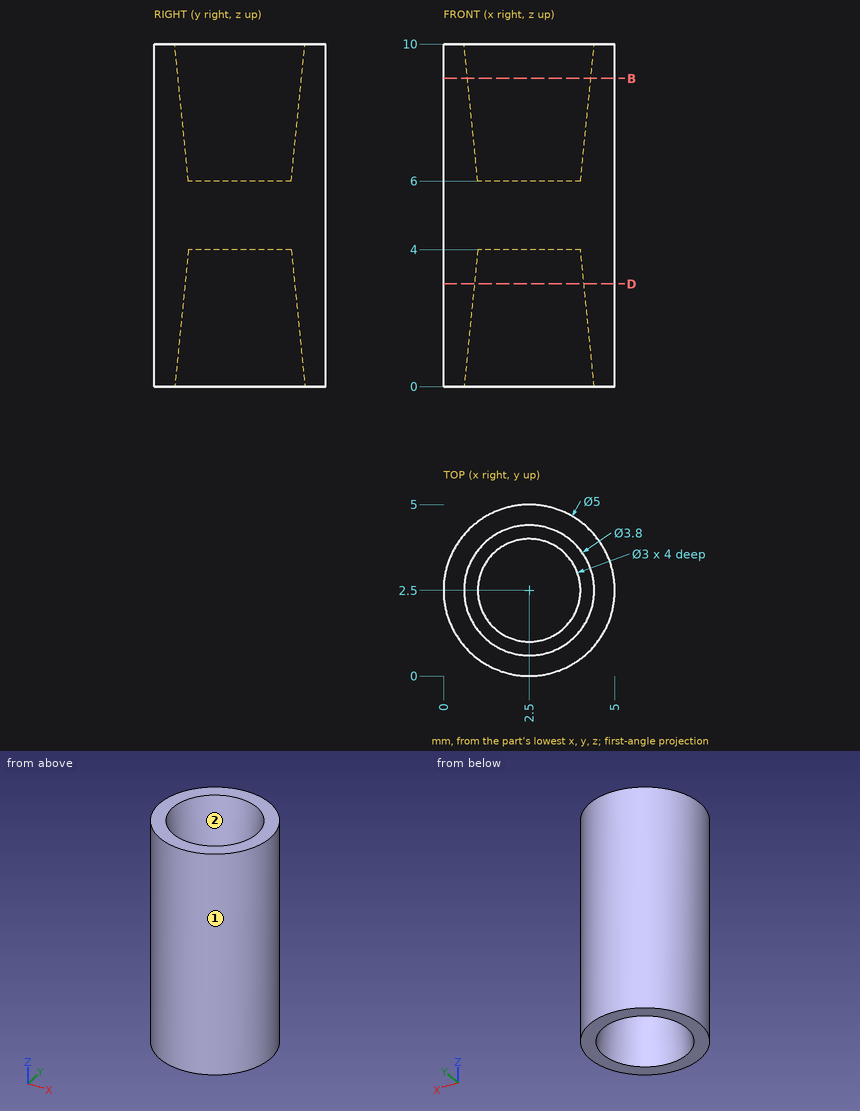
Part print with two shaded views. Sizes in mm from the minimum x, y, z corner. Round coordinates to 2 decimals unless told otherwise and drop trailing zeros. Loops run counter-clockwise (first coordinate to the right, second up) from the corner with the lowest first, then second, coordinate; pieces in that order, holes last. Notation, with made-up numbers: (-33, 9) - (17, 9) arc R17 cw to (17, 41) - close; hole circle Ø2 at (-10.5, 46). An arc over 180 degrees is marked (long way). Answer as a JSON object with one key per item and string values.
Item 1: Band-saw the part on D-D on z = 3. List the corners of the cut face in (x, y).
Output:
{"outline": "circle Ø5 at (2.5, 2.5); hole circle Ø3.2 at (2.5, 2.5)"}
Item 2: Pull direction Y, two halves, no side cores. Call the marked faces 1 and 2: pulls with the +Y half, pulls with the -Y half, needs draft (parallel to the pull), parting line crosses it, or undercut.
Output:
{"face 1": "parting line crosses it", "face 2": "undercut"}
Item 3: Band-saw the part on B-B on z = 9. List the corners of the cut face in (x, y).
Output:
{"outline": "circle Ø5 at (2.5, 2.5); hole circle Ø3.6 at (2.5, 2.5)"}
Item 4: Pin check, flat tips, straight feed: pin 1 (3 mm diameter, centred on x = 1, y = 2.5, fed in from -Z); pin 2 (0.9 mm diameter, centred on x = 3, y = 3, fed in from +Z); pin 3 (1.5 mm diameter, centred on x = 1, z = 2, fed in from -Y); pin 4 (1.5 mm diameter, centred on x = 3, y = 2, fed in from -Z). Stop position of each tip, or through.
Output:
{"pin 1": "z = 0", "pin 2": "z = 6", "pin 3": "y = 0.12", "pin 4": "z = 4"}
Item 5: Wall check: L1, parallel to Z at x = 3.55, y = 2.75; L2, parallel to Y at x = 0.5, z = 7.25; L3, parallel to X at y = 3.1, z = 8. Give the ranges that are in metal, low to high.
Output:
{"L1": "4 to 6", "L2": "1 to 4", "L3": "0.07 to 0.91, 4.09 to 4.93"}
